Geometry: final body of the model. Coordinates: model frame, mm. A direction names the side the tool comes from. Give positions to 0.01 mm unless a question says otherwise; leave off trailing zeros. Write each loop counter-clockwise with the first axis right and the second up, starting at its lowest first coordinate (ties: lowest second). Pieces come first, ordered by that corner, then holes. Notation, with made-up numbers: (-37.75, 61.5) -> (-11.75, 61.5) arc R24 ccw to (-11.75, 77.5) -> close; hole circle Ø7 at (84.25, 88). An arc over 180 degrees is marked (long way). Answer in a Markdown table with one row per item. Add a question column.
Item 1: Access query for faces 4 (the conical face through (0.3, -13.9, 1.9)), 5 (the flat face through (0, 0, 0)), 6 (the flat face through (-15, -3, 3)). Directions: +Z, -Z, +X, -X, +Y, -Y. A direction counts if a zero-diameter tool reaches every point of the face in a straight line with its end or side. Return the directions, or none.
Item 2: First-contact query: P1, Ø1.2, axis at x = -15, z = 3.5, coming from the +Y side; P2, Ø2, axis at x = -15.5, z = 4.5, coming from the -Y side; P3, Ø3, axis at x = -9, z = 2, coming from the +Y side. Flat tips, straight axial feed; report the tip coordinate or a pass-through.
Item 3: Section query C-C on y = 0. Output: boundary loops of the cut face in (x, z), plus the area to 3 significant figures.
Item 4: Section query A-A on x = 0. Output: boundary loops of the cut face in (y, z), plus the area to 3 significant figures.
Item 5: Section query D-D on z = 2.5. Output: boundary loops of the cut face in (x, y), plus the area to 3 significant figures.
Item 6: Section query B-B on z = 4.5. Output: boundary loops of the cut face in (x, y), plus the area to 3 significant figures.
Item 7: Material intervals for probe 1 along X at (y, z) = (-5, 4.25); probe 2 along X at (y, z) = (5, 1.25); probe 3 along Y at (x, z) = (11.5, 2.5), sorted ascending. Write a range as from..to.
Item 8: Draft query along Y for faces 1 (the flat face through (0.1, 16.5, 6)), 2 (the conical face through (-12.604, 6.555, 0.375)), 3 (the flat face through (0, 0, 1)). Return one class per face: +Y half, -Y half, draft (parallel to the pull), parting line (faces both ways), or undercut.
```python
from build123d import *

# Parameters (mm, degrees)
F2_T     = -1
F4_DEPTH = 5.001


with BuildPart() as f1:
    # F0 (on Right) → F1 (revolve)
    with BuildSketch(Plane.YZ):
        Polygon((0, 6), (0, 0), (14, 0), (17.3028167337, 6), align=None)
    revolve(axis=Axis((0, 0, 3), (0, 0, -1)))

    # F2
    f2_openings = [f1.faces().sort_by_distance(p)[0] for p in [
        (0, 0, 6),
    ]]
    offset(amount=F2_T, openings=f2_openings)

    # F3 (on face) → F4 (cut, through all)
    with BuildSketch(Plane.XY.offset(1)):
        with BuildLine():
            Line((13.0690676017, -3), (25, -3))
            Line((25, -3), (25, 3))
            Line((25, 3), (13.0690676017, 3))
            ThreePointArc((13.0690676017, 3), (13.3237248636, 1.50959721), (13.408971921, 0))
            ThreePointArc((13.408971921, 0), (13.3237248636, -1.50959721), (13.0690676017, -3))
        make_face()
        with BuildLine():
            Line((-25, -3), (-13.0690676017, -3))
            ThreePointArc((-13.0690676017, -3), (-13.408971921, 0), (-13.0690676017, 3))
            Line((-13.0690676017, 3), (-25, 3))
            Line((-25, 3), (-25, -3))
        make_face()
        with BuildLine():
            Line((-13.0690676017, -3), (13.0690676017, -3))
            ThreePointArc((13.0690676017, -3), (13.3237248636, -1.50959721), (13.408971921, 0))
            ThreePointArc((13.408971921, 0), (13.3237248636, 1.50959721), (13.0690676017, 3))
            Line((13.0690676017, 3), (-13.0690676017, 3))
            ThreePointArc((-13.0690676017, 3), (-13.408971921, 0), (-13.0690676017, -3))
        make_face()
    extrude(amount=F4_DEPTH, mode=Mode.SUBTRACT)


solid = f1.part
```
Findings below:
| question | item | result |
|---|---|---|
| 1 | face 4 | +Z |
| 1 | face 5 | -Z, +X, -X, +Y, -Y |
| 1 | face 6 | +Z, +X, -X |
| 2 | P1 | stops at y = 7.02 |
| 2 | P2 | stops at y = -8.16 |
| 2 | P3 | stops at y = 13.53 |
| 3 | outline | (-14.55, 1) -> (-14, 0) -> (14, 0) -> (14.55, 1) -> close |
| 3 | area | 28.6 mm^2 |
| 4 | outline | (-17.3, 6) -> (-14, 0) -> (14, 0) -> (17.3, 6) -> (16.16, 6) -> (13.41, 1) -> (-13.41, 1) -> (-16.16, 6) -> close |
| 4 | area | 40.0 mm^2 |
| 5 | outline | (-15.08, -3) arc R15.38 ccw to (15.08, -3) -> (13.91, -3) arc R14.23 cw to (-13.91, -3) -> close; (-15.08, 3) -> (-13.91, 3) arc R14.23 cw to (13.91, 3) -> (15.08, 3) arc R15.38 ccw to start |
| 5 | area | 92.4 mm^2 |
| 6 | outline | (-16.2, -3) arc R16.48 ccw to (16.2, -3) -> (15.04, -3) arc R15.34 cw to (-15.04, -3) -> close; (-16.2, 3) -> (-15.04, 3) arc R15.34 cw to (15.04, 3) -> (16.2, 3) arc R16.48 ccw to start |
| 6 | area | 100 mm^2 |
| 7 | probe 1 | x = -15.56..-14.35, 14.35..15.56 |
| 7 | probe 2 | x = -13.81..-12.59, 12.59..13.81 |
| 7 | probe 3 | y = -10.21..-8.39, 8.39..10.21 |
| 8 | face 1 | draft |
| 8 | face 2 | parting line |
| 8 | face 3 | undercut |
